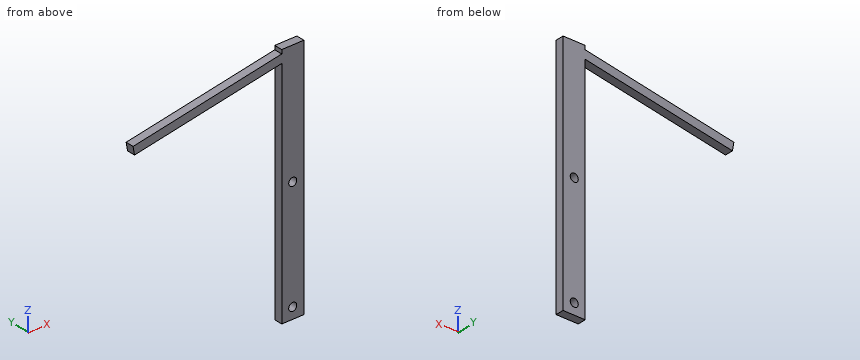
```python
from build123d import *

# Parameters (mm, degrees)
SKETCH1_W           = 12.7
SKETCH1_H           = 139.7
SKETCH1_R           = 2.31
BOSS_EXTRUDE1_DEPTH = 4.7625
BOSS_EXTRUDE2_DEPTH = 4.7625


with BuildPart() as part:
    # Sketch1 → Boss-Extrude1 (new body)
    with BuildSketch(Plane(origin=(0, 0, 0), x_dir=(1, 0, 0), z_dir=(0, 1, 0))):
        with Locations((6.35, 31.687542426)):
            Rectangle(SKETCH1_W, SKETCH1_H)
        with Locations(Location((6.293214881, 95.187542426, 0), (0, 0, 90))):
            Circle(SKETCH1_R, mode=Mode.SUBTRACT)
        with Locations(Location((6.293214881, 31.537542426, 0), (0, 0, 90))):
            Circle(SKETCH1_R, mode=Mode.SUBTRACT)
    extrude(amount=BOSS_EXTRUDE1_DEPTH)

    # Sketch2 → Boss-Extrude2 (add)
    with BuildSketch(Plane.XZ):
        Polygon((0, 31.08713568), (0, 35.923104919), (-85.288371425, 20.884463896), (-84.461371979, 16.194316973), align=None)
    extrude(amount=-BOSS_EXTRUDE2_DEPTH)


solid = part.part
```
The listing builds one solid part. Answer for the finished solid, in the listing's coordinates (mm). Coordinates: 2 decimals unless noted, no trailing zeros. Write each loop counter-clockwise with the first axis right and the second up, starting at its lowest first coordinate (ties: lowest second). Pieces come first, ordered by that corner, then holes. Notation, with made-up numbers: (53.25, 5.5) - (71.25, 5.5) arc R22 ccw to (71.25, 39.5) - close; hole circle Ø3 at (46, 45.5). An arc over 180 degrees is marked (long way). Return JSON: item names as keys, results as strings. Group by question number.
1. Straight lines are drawn through the part: L1, parallel to Z at x = 7.5, y = 3.8; L2, parallel to X at y = 2.8, z = -36.5; L3, parallel to Z at x = 4.5, y = 1.15. For each, find the intervals that lie inside material, in ascending order.
2. Given pin 1 (2.5 mm diameter, centred on y = 1.5, z = -16.5, fed in from -X); pin 2 (3.5 mm diameter, centred on x = 6.29, z = -31.54, fed in from +Y), each flat-ended and moving along its own axis, determine where each tip first touches the part or whether it passes through.
3. A cutting plane is placed at D-D, the plane x = -67.5. Determine the outline of the cut face in (y, z), plus the area to 3 significant figures.
4. A cutting plane is placed at A-A, the plane z = 22.5. Determine the outline of the cut face in (x, y), plus the area to 3 significant figures.
5. A cutting plane is placed at B-B, the plane y = 2. Determine the outline of the cut face in (x, z).
6. A cutting plane is placed at C-C, the plane z = -87.5. Determine the outline of the cut face in (x, y).
Ans:
{
 "1": {"L1": "-101.54 to -97.16, -93.22 to -33.51, -29.57 to 38.16", "L2": "0 to 12.7", "L3": "-101.54 to -96.64, -93.73 to -32.99, -30.08 to 38.16"},
 "2": {"pin 1": "x = 0", "pin 2": "through"},
 "3": {"outline": "(0, 19.19) - (4.76, 19.19) - (4.76, 24.02) - (0, 24.02) - close", "area": "23.0 mm²"},
 "4": {"outline": "(-76.13, 0) - (-48.7, 0) - (-48.7, 4.76) - (-76.13, 4.76) - close; (0, 0) - (12.7, 0) - (12.7, 4.76) - (0, 4.76) - close", "area": "191 mm²"},
 "5": {"outline": "(-85.29, 20.88) - (-84.46, 16.19) - (0, 31.09) - (0, -101.54) - (12.7, -101.54) - (12.7, 38.16) - (0, 38.16) - (0, 35.92) - close; hole circle Ø4.62 at (6.29, -95.19); hole circle Ø4.62 at (6.29, -31.54)"},
 "6": {"outline": "(0, 0) - (12.7, 0) - (12.7, 4.76) - (0, 4.76) - close"}
}
